from build123d import *

# Parameters (mm, degrees)
F1_DEPTH = 127
F2_R     = 5.518892


with BuildPart() as f1:
    # F0 (on Front) → F1 (new body)
    with BuildSketch(Plane.XZ):
        with BuildLine():
            Line((62.236424, 50.8), (-64.763576, 50.8))
            Line((-64.763576, 50.8), (-64.763576, 0))
            Line((-64.763576, 0), (-50.493699, 0))
            ThreePointArc((-50.493699, 0), (-25.246849, 22.614934), (0, 0))
            ThreePointArc((0, 0), (25.229008, 22.457695), (50.458016, 0))
            Line((50.458016, 0), (62.236424, 0))
            Line((62.236424, 0), (62.236424, 50.8))
        make_face()
    extrude(amount=F1_DEPTH)

    # F2
    f2_edges = [f1.edges().sort_by_distance(p)[0] for p in [
        (-1.263576, 0, 50.8),
        (-64.763576, -63.5, 50.8),
        (-1.263576, -127, 50.8),
        (62.236424, -63.5, 50.8),
    ]]
    fillet(f2_edges, radius=F2_R)


solid = f1.part
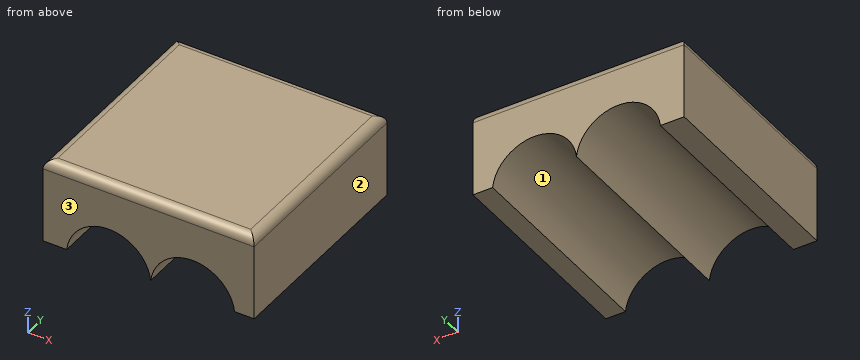
Work out the finished part from the listing and answer in its coordinate system (mm). Face numbers are marked on the shaded views. Round coordinates to 2 decimals unless told otherwise and drop trailing zeros. Order: outer loops, then holes, each group sorted by start corner. A loop starts at its lowest first (then second) coordinate and runs counter-clockwise, first axis right, second up. Notation, with made-up numbers: M 41.5,-30.5 L 77.5,-30.5 A9 cw 77.5,-25.5 Z; hole C 11,58.25 d11. An arc over 180 degrees is marked long. One line per item, written item: value.
Q1. Find section C-C on x = -3.5. Write down the section's boundary in (y, z).
Derived:
outline: M -127,10.34 L 0,10.34 L 0,45.28 A5.52 ccw -5.52,50.8 L -121.48,50.8 A5.52 ccw -127,45.28 Z
Q2. Straight lines are drawn through the part: line 1 (X direction, y = -78, z = 10); line 2 (X direction, y = -72.5, z = 16); line 3 (Y direction, x = 50, z = 49). For each, find the intervals that lie inside material, in ascending order.
Derived:
line 1: -64.76 to -47.19, -3.3 to 3.37, 47.08 to 62.24
line 2: -64.76 to -42.34, -8.15 to 8.31, 42.15 to 62.24
line 3: -125.56 to -1.44
Q3. Find section D-D on x = 44.5. Write down the section's boundary in (y, z).
Derived:
outline: M -127,13.6 L 0,13.6 L 0,45.28 A5.52 ccw -5.52,50.8 L -121.48,50.8 A5.52 ccw -127,45.28 Z
Q4. Find section A-A on z = 3.5. Write down the section's boundary in (x, y), then the cut area to 3 significant figures.
Derived:
outline: M -64.76,-127 L -49.86,-127 L -49.86,0 L -64.76,0 Z; M -0.64,-127 L 0.66,-127 L 0.66,0 L -0.64,0 Z; M 49.8,-127 L 62.24,-127 L 62.24,0 L 49.8,0 Z
area: 3,640 mm²
Q5. A flat-ended cylindrical pin translates along its axis: pin 1 (8 mm diameter, centred on x = 39, y = -79.5, fed in from -Z). Find the tip coordinate at first contact, or state that the pin passes through.
Derived:
pin 1: z = 15.21
Q6. Find section B-B on y = -41.5. Write down the section's boundary in (x, z).
Derived:
outline: M -64.76,0 L -50.49,0 A25.4 cw 0,0 A25.4 cw 50.46,0 L 62.24,0 L 62.24,45.28 A5.52 ccw 56.72,50.8 L -59.24,50.8 A5.52 ccw -64.76,45.28 Z
Q7. Determine the mould class of the marked faces 1, 2 and 3 for opening direction X: released by +X, released by -X, zero draft, split by the parting line, or undercut.
Derived:
face 1: undercut
face 2: released by +X
face 3: zero draft
